Geometry check sheet. Reference: the model listing, model coordinates, mm. A direction names the side the tool comes from. Coordinates: 2 decimals unless noted, no trailing zeros. Loops run counter-clockwise (first coordinate to the right, second up) from the corner with the lowest first, then second, coordinate; pieces in that order, holes last. Notation, with made-up numbers: (-13.75, 53) - (38.25, 53) arc R18 cw to (38.25, 73) - close; hole circle Ø11 at (34.5, 86). An arc over 180 degrees is marked (long way). One line per item, written item: value.
from build123d import *

# Parameters (mm, degrees)
HEX_2_DEPTH = 1.5


with BuildPart() as part:
    # BodySke → BaseBody (revolve)
    with BuildSketch(Plane.XY, mode=Mode.PRIVATE) as basebody_sk:
        Polygon((0, 0), (0, 1.61), (0.225166605, 2), (4.845299462, 2), (6, 0), align=None)
    revolve(basebody_sk.sketch.rotate(Axis((-12.7, 0, 0), (1, 0, 0)), 90), axis=Axis((-12.7, 0, 0), (1, 0, 0)))  # turned: the seam where the file's is

    # Sketch2 → Hex 2 (cut)
    with BuildSketch(Plane.ZY):
        Polygon((0.577350269, 1), (-0.577350269, 1), (-1.154700538, 0), (-0.577350269, -1), (0.577350269, -1), (1.154700538, 0), align=None)
    extrude(amount=-HEX_2_DEPTH, mode=Mode.SUBTRACT)


solid = part.part
(1) Cross-section at A-A on x = 1.3. Record the cut outline in (y, z).
Reply:
outline: circle Ø4 at (0, 0); hole (-1, -0.58) - (0, -1.15) - (1, -0.58) - (1, 0.58) - (0, 1.15) - (-1, 0.58) - close
(2) Cross-section at B-B on x = 3.1. Record the cut outline in (y, z).
Reply:
outline: circle Ø4 at (0, 0)
(3) Cross-section at C-C on x = 5.05. Record the cut outline in (y, z).
Reply:
outline: circle Ø3.29 at (0, 0)
(4) Material ranges on probe 1 along Z at (x, y) = (0.75, 0.5); probe 2 along Y at (x, z) = (1.05, -0.45); probe 3 along X at (y, z) = (-1.15, -1.3), recorded low to high. Write a range as from..to.
Reply:
probe 1: -1.94..-0.87, 0.87..1.94
probe 2: -1.95..-1, 1..1.95
probe 3: 0.07..5
(5) Release check for a two-part mould opening along Z. For faces 1 (the face through (0.74, 0.51, -0.86)), 2 (the face through (0, -1, 1)), 3 (the face through (3, 2, 0)) record: pulls with the +Z half, pulls with the -Z half, needs draft (parallel to the pull), parting line crosses it, or undercut.
Reply:
face 1: undercut
face 2: needs draft
face 3: parting line crosses it
(6) Go/stop test with flat-tipped pins: pin 1 Ø2 at (x, y) = (1, -1.5) entering from +Z; pin 2 Ø2 at (x, z) = (3, 1.5) entering from +Y. Record where each tip stops, or that it passes through.
Reply:
pin 1: z = 1.94
pin 2: y = 1.94
(7) Access from +Z, -Z, +X, -X, +Y, -Y to the whole of each face (thin tool, end or side, straight path). Record for faces 4 (the face through (0.74, -0.49, -0.87)), 5 (the face through (6, 0, 0)).
Reply:
face 4: -X
face 5: +X
